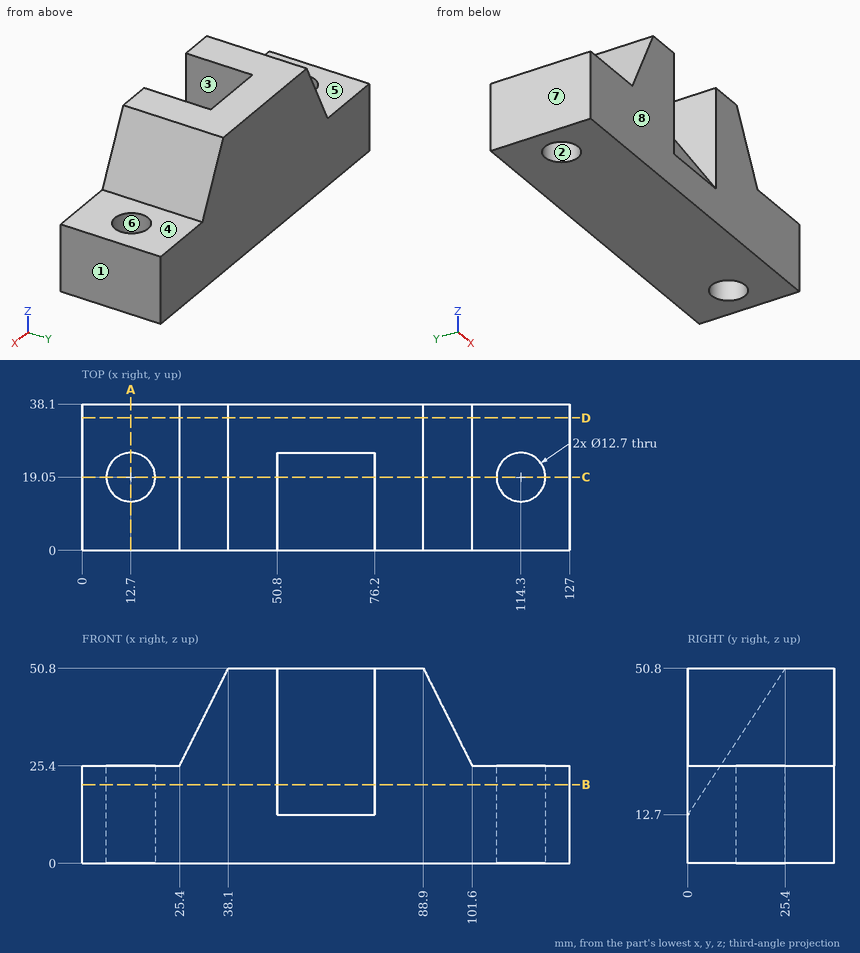
Study the drawing (mm; zero at the part's minimum x, y, z) and answer. A direction names the side the tool comes from. Round coordinates to 2 decimals unless told otherwise and drop trailing zeros. Write each loop counter-clockwise with the first axis right and the second up, starting at its lowest first coordinate (ties: lowest second). Pieces come first, ordered by that corner, then holes.
1) Straight lines are drawn through the part: line 1 (X direction, y = 19, z = 16); line 2 (Y direction, x = 114, z = 11); line 3 (Z direction, x = 103, y = 12.5). For each, find the intervals that lie inside material, in ascending order.
2) The mould has two halves that part along Y. Classify the marked faces 6, 7 and 8: pulls with the +Y half, pulls with the -Y half, needs draft (parallel to the pull), parting line crosses it, or undercut.
3) A cutting plane is placed at B-B (z = 20.5). Give the vertices of the cut face in (x, y).
4) A tool of negligible diameter and unlimited length cuts with its end or side. For the marked faces 1, 2, 3, 4 and 5, from which of +Z, -Z, +X, -X, +Y, -Y can it reach the whole face along a straight path? Write none if from no direction.
5) A cutting plane is placed at D-D (y = 34.5). Give the vertices of the cut face in (x, z), plus the area to 3 significant figures.
6) A cutting plane is placed at A-A (x = 12.7). Give the vertices of the cut face in (y, z).
7) A cutting plane is placed at C-C (y = 19.05). Give the vertices of the cut face in (x, z) (3 decimals).
8) Given pin 1 Ø1 at (y, z) = (29.5, 34) entering from -X; pin 2 Ø8 at (x, y) = (15.5, 22) entering from +Z; pin 3 Ø20.5 at (x, y) = (17, 21) entering from +Z, each flat-ended and moving along its own axis, determine where each tip first touches the part or whether it passes through.
Completed:
1. line 1: x = 0 to 6.35, 19.05 to 107.95, 120.65 to 127
1. line 2: y = 0 to 12.71, 25.39 to 38.1
1. line 3: z = 0 to 25.4
2. face 6: undercut
2. face 7: needs draft
2. face 8: pulls with the -Y half
3. outline: (0, 0) - (50.8, 0) - (50.8, 5.2) - (76.2, 5.2) - (76.2, 0) - (127, 0) - (127, 38.1) - (0, 38.1) - close; hole circle Ø12.7 at (12.7, 19.05); hole circle Ø12.7 at (114.3, 19.05)
4. face 1: +Z, -Z, +X, +Y, -Y
4. face 2: +Z, -Z
4. face 3: +Z, -Y
4. face 4: +Z, +X, +Y, -Y
4. face 5: +Z, -X, +Y, -Y
5. outline: (0, 0) - (127, 0) - (127, 25.4) - (101.6, 25.4) - (88.9, 50.8) - (38.1, 50.8) - (25.4, 25.4) - (0, 25.4) - close
5. area: 4,840 mm2
6. outline: (0, 0) - (12.7, 0) - (12.7, 25.4) - (0, 25.4) - close; (25.4, 0) - (38.1, 0) - (38.1, 25.4) - (25.4, 25.4) - close
7. outline: (0, 0) - (6.35, 0) - (6.35, 25.4) - (0, 25.4) - close; (19.05, 0) - (107.95, 0) - (107.95, 25.4) - (101.6, 25.4) - (88.9, 50.8) - (76.2, 50.8) - (76.2, 41.275) - (50.8, 41.275) - (50.8, 50.8) - (38.1, 50.8) - (25.4, 25.4) - (19.05, 25.4) - close; (120.65, 0) - (127, 0) - (127, 25.4) - (120.65, 25.4) - close
8. pin 1: stops at x = 29.45
8. pin 2: stops at z = 25.4
8. pin 3: stops at z = 29.1
